The model under review builds one solid part; all positions refer to its coordinate system, in mm. Face numbers are marked on the shaded views. Coordinates: 2 decimals unless noted, no trailing zeros. Order: outer loops, then holes, each group sorted by start corner. A loop starts at its lowest first (then second) coordinate and runs counter-clockwise, first axis right, second up. Notation, with made-up numbers: (58.25, 7.25) -> (96.25, 7.25) arc R22 ccw to (96.25, 27.25) -> close; hole circle Ø11 at (81, 71.25). An arc over 180 degrees is marked (long way). Use CSV: the item, a comma, the result in double quotes. Start each with the question number.
Autodesk Inventor part; units mm, degrees
ref_plane "YZ Plane" through (0, 0, 0) normal (1, 0, 0) x (0, 1, 0)
ref_plane "XZ Plane" through (0, 0, 0) normal (0, 1, 0) x (-1, 0, 0)
ref_plane "XY Plane" through (0, 0, 0) normal (0, 0, 1) x (1, 0, 0)
sketch "Sketch1" plane through (0, 0, 0) normal (0, 1, 0) x (-1, 0, 0)
  circle A0 centre (0, 0) radius 7.75
  circle A1 centre (0, 0) radius 9.75
  dimension "d0" = 15.5
  dimension "d1" = 19.5
extrude "Extrusion1" add sketch "Sketch1" along normal blind 5.5
sketch "Sketch5" plane through (0, 5.5, 0) normal (0, 1, 0) x (1, 0, 0)
  circle A0 centre (0, 0) radius 10.5
  circle A1 centre (0, 0) radius 8.75
  dimension "d14" = 21
  dimension "d15" = 17.5
extrude "Extrusion5" add sketch "Sketch5" along normal blind 3
fillet "Fillet1" radius 2 1 edges at (-8.75, 5.5, 0)
move faces "Move1" translate (0, -0.5, 0) faces at (10.0539, 5.5, 1.6154)
properties part number "685ZZFlanged_Adapter"
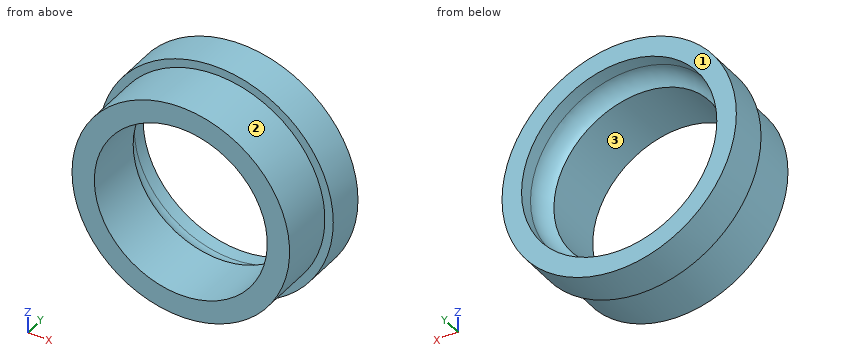
Q1. To check wall thickness, follow probe 1 along Z at (x, y) = (0, 3.25); probe 2 along Z at (x, y) = (0, 8.15); probe 3 along X at (y, z) = (6.75, -4). State the ranges of each line that lie inside material, in increasing order.
Q2. Add section B-B, the plane x = 0. State the section outline as (y, z) points, then the cut area to 3 significant figures.
Q3. Draft analysis for pull direction X (two halves, no side actions). For the marked faces 1, 2 and 3, state which applies: +X half, -X half, draft (parallel to the pull), parting line (faces both ways), or undercut.
Q4. Add section C-C, the plane y = 7.5. State the section outline as (x, z) points.
Q5. Add section D-D, the plane z = 9. State the section outline as (x, y) points, then the cut area to 3 significant figures.
Q6. Add section A-A, the plane z = 0. State the section outline as (x, y) points.
Answer block:
1,probe 1,"z = -9.75 to -7.75, 7.75 to 9.75"
1,probe 2,"z = -10.5 to -8.75, 8.75 to 10.5"
1,probe 3,"x = -9.71 to -7.72, 7.72 to 9.71"
2,outline,"(0, -9.75) -> (5, -9.75) -> (5, -10.5) -> (8.5, -10.5) -> (8.5, -8.75) -> (7.23, -8.75) arc R2 cw to (5.5, -7.75) -> (0, -7.75) -> close; (0, 7.75) -> (5.5, 7.75) arc R2 cw to (7.23, 8.75) -> (8.5, 8.75) -> (8.5, 10.5) -> (5, 10.5) -> (5, 9.75) -> (0, 9.75) -> close"
2,area,"34.3 mm²"
3,face 1,"draft"
3,face 2,"parting line"
3,face 3,"undercut"
4,outline,"circle Ø21 at (0, 0); hole circle Ø17.5 at (0, 0)"
5,outline,"(-5.41, 5) -> (-3.75, 5) -> (-3.75, 0) -> (3.75, 0) -> (3.75, 5) -> (5.41, 5) -> (5.41, 8.5) -> (-5.41, 8.5) -> close"
5,area,"75.4 mm²"
6,outline,"(-10.5, 5) -> (-9.75, 5) -> (-9.75, 0) -> (-7.75, 0) -> (-7.75, 5.5) arc R2 cw to (-8.75, 7.23) -> (-8.75, 8.5) -> (-10.5, 8.5) -> close; (7.75, 0) -> (9.75, 0) -> (9.75, 5) -> (10.5, 5) -> (10.5, 8.5) -> (8.75, 8.5) -> (8.75, 7.23) arc R2 cw to (7.75, 5.5) -> close"
